from build123d import *

# Parameters (mm, degrees)
F0_R     = 47.625
F0_R_2   = 12.7
F1_DEPTH = 9.525
F2_W     = 23.8125
F2_H     = 10
F3_DEPTH = 9.526
F4_SIZE  = 1.5875


with BuildPart() as f1:
    # F0 (on Top) → F1 (new body)
    with BuildSketch(Plane.XY):
        Circle(F0_R)
        Circle(F0_R_2, mode=Mode.SUBTRACT)
    extrude(amount=F1_DEPTH)

    # F2 (on face) → F3 (cut, through all)
    with BuildSketch(Plane.XY.offset(9.525)):
        with Locations((-28.479498, 0)):
            Rectangle(F2_W, F2_H)
        Polygon((-12.616751, 11.852853), (-3.956497, 16.852853), (-15.862747, 37.475083), (-24.523001, 32.475083), align=None)
        Polygon((3.956497, 16.852853), (12.616751, 11.852853), (24.523001, 32.475083), (15.862747, 37.475083), align=None)
        with Locations((28.479498, 0)):
            Rectangle(F2_W, F2_H)
        Polygon((12.616751, -11.852853), (3.956497, -16.852853), (15.862747, -37.475083), (24.523001, -32.475083), align=None)
        Polygon((-3.956497, -16.852853), (-12.616751, -11.852853), (-24.523001, -32.475083), (-15.862747, -37.475083), align=None)
    extrude(amount=-F3_DEPTH, mode=Mode.SUBTRACT)

    # F4
    f4_edges = [f1.edges().sort_by_distance(p)[0] for p in [
        (-28.479498, 5, 9.525),
        (-40.385748, 0, 9.525),
        (-28.479498, -5, 9.525),
        (-16.573248, 0, 9.525),
        (-12.7, 0, 9.525),
        (-8.286624, 14.352853, 9.525),
        (-18.569876, 22.163968, 9.525),
        (-9.909622, 27.163968, 9.525),
        (-20.192874, 34.975083, 9.525),
        (9.909622, 27.163968, 9.525),
        (20.192874, 34.975083, 9.525),
        (8.286624, 14.352853, 9.525),
        (18.569876, 22.163968, 9.525),
        (16.573248, 0, 9.525),
        (28.479498, 5, 9.525),
        (40.385748, 0, 9.525),
        (28.479498, -5, 9.525),
        (18.569876, -22.163968, 9.525),
        (8.286624, -14.352853, 9.525),
        (9.909622, -27.163968, 9.525),
        (20.192874, -34.975083, 9.525),
        (-9.909622, -27.163968, 9.525),
        (-20.192874, -34.975083, 9.525),
        (-18.569876, -22.163968, 9.525),
        (-8.286624, -14.352853, 9.525),
        (-47.625, 0, 9.525),
    ]]
    chamfer(f4_edges, length=F4_SIZE)


solid = f1.part
The model under review builds one solid part; all positions refer to its coordinate system, in mm. A direction names the side the tool comes from. Round coordinates to 2 decimals unless told otherwise and drop trailing zeros. Order: outer loops, then holes, each group sorted by start corner. A loop starts at its lowest first (then second) coordinate and runs counter-clockwise, first axis right, second up. Notation, with made-up numbers: (73, 86) -> (80, 86) arc R26 ccw to (80, 112) -> close; hole circle Ø2 at (39.25, 1.25). An arc over 180 degrees is marked (long way). Return JSON: item names as keys, results as strings.
1. The part is to be moulded in two halves that separate along X. For faces 1 (the face through (10, -10, 0)), 2 (the face through (9.826, -27.02, 4.024)), say which applies: +X half, -X half, draft (parallel to the pull), parting line (faces both ways), or undercut.
Answer block:
{"face 1": "draft", "face 2": "undercut"}
2. Take a section at C-C (z = 3.5). State how many separate pieces and enclosed holes the cut face has, then the cut area to 3 significant figures.
Answer block:
{"separate pieces": "1", "enclosed holes": "7", "area": "5,190 mm²"}
3. Take a section at A-A (x = 0). Write out the cut boundary in (y, z) (1 decimal), then the cut area to 3 significant figures.
Answer block:
{"outline": "(-47.6, 0) -> (-12.7, 0) -> (-12.7, 7.9) -> (-14.3, 9.5) -> (-46, 9.5) -> (-47.6, 7.9) -> close; (12.7, 0) -> (47.6, 0) -> (47.6, 7.9) -> (46, 9.5) -> (14.3, 9.5) -> (12.7, 7.9) -> close", "area": "660 mm²"}
4. Insertion check: P1, Ø2, axis at x = -18.5, z = 4, coming from the +Y side; P2, Ø5, axis at x = 24, z = 3, coming from the +Y side; P3, Ø4, axis at y = 2, z = 5.5, coming from the -X side (3 decimals); P4, Ø2, axis at x = -21.5, y = 31.5, coming from the +Z side. Each pin has a flat end and moves straight along its axis. Give the tip position at first contact, or say it passes through.
Answer block:
{"P1": "stops at y = 44.29", "P2": "stops at y = 42.5", "P3": "stops at x = -47.625", "P4": "passes through"}
5. For L1, parallel to X at y = 1.5, z = 2.75; L2, parallel to Y at x = 9, z = 4; L3, parallel to Y at x = -16, z = 1.25, list the stretches that pass through material, from the lowest coordinate up. Write a range as [from, to].
Answer block:
{"L1": "x = [-47.6, -40.39], [-16.57, -12.61], [12.61, 16.57], [40.39, 47.6]", "L2": "y = [-46.77, -25.59], [-13.94, -8.96], [8.96, 13.94], [25.59, 46.77]", "L3": "y = [-44.86, -37.4], [-17.71, 17.71], [37.4, 44.86]"}
6. Take a section at B-B (y = 0). Write out the cut boundary in (x, z) (1 decimal), then the cut area to 3 significant figures.
Answer block:
{"outline": "(-47.6, 0) -> (-40.4, 0) -> (-40.4, 7.9) -> (-42, 9.5) -> (-46, 9.5) -> (-47.6, 7.9) -> close; (-16.6, 0) -> (-12.7, 0) -> (-12.7, 7.9) -> (-14.3, 9.5) -> (-15, 9.5) -> (-16.6, 7.9) -> close; (12.7, 0) -> (16.6, 0) -> (16.6, 7.9) -> (15, 9.5) -> (14.3, 9.5) -> (12.7, 7.9) -> close; (40.4, 0) -> (47.6, 0) -> (47.6, 7.9) -> (46, 9.5) -> (42, 9.5) -> (40.4, 7.9) -> close", "area": "202 mm²"}
7. For faces 3 (the face through (7.82, 13.72, 8.72)), 4 (the face through (18.653, -22.308, 4.024)), list the 3-axis set-ups (+Z, -Z, +X, -X, +Y, -Y) from which the entire face can be reached by the end or side of a thin tool; tool diameter is ignored.
Answer block:
{"face 3": "+Z", "face 4": "+Z, -Z"}
